from build123d import *

# Parameters (mm, degrees)
TALADRO_DE_MARGEN_PARA_1_41_D = 6.7564


with BuildPart() as part:
    # Croquis2 → Revolución1 (revolve)
    with BuildSketch(Plane.XY, mode=Mode.PRIVATE) as revoluci_n1_sk:
        Polygon((9.5, 37.5), (9.5, -37.5), (13.5, -37.5), (13.5, -7.5), (25.4, -7.5), (25.4, 7.5), (13.5, 7.5), (13.5, 37.5), align=None)
    revolve(revoluci_n1_sk.sketch.rotate(Axis((0, 0, 0), (0, -1, 0)), 90), axis=Axis((0, 0, 0), (0, -1, 0)))

    # Taladro de margen para 1/41 (through all)
    with Locations(Plane(origin=(0, 7.5, 0), x_dir=(1, 0, 0), z_dir=(0, 1, 0))):
        with Locations((19.45, 0), (-19.45, 0)):
            Hole(TALADRO_DE_MARGEN_PARA_1_41_D / 2)


solid = part.part
Source: CAD feature listing. Evaluate the final solid. Frame: model axes, mm. A direction names the side the tool comes from. Round coordinates to 2 decimals unless told otherwise and drop trailing zeros. Loops run counter-clockwise (first coordinate to the right, second up) from the corner with the lowest first, then second, coordinate; pieces in that order, holes last. Notation, with made-up numbers: (84.25, 39) - (95.25, 39) arc R9 cw to (95.25, 55) - close; hole circle Ø6 at (47, -17). An arc over 180 degrees is marked (long way). Write item = value, one per line. Start each with the question number.
(1) Pin query (flat end, axial travel): pin 1 (3 mm diameter, centred on y = 0.5, z = 20, fed in from +X); pin 2 (10 mm diameter, centred on x = -1.5, y = 17.5, fed in from -Z); pin 3 (8 mm diameter, centred on x = 19.45, z = 0, fed in from -Y); pin 4 (8 mm diameter, centred on x = 2.5, z = 7.5, fed in from -Y). Return the tip coordinate at first contact, or that it passes through.
(2) Pull-direction query (Z, two-part tool) for faces 4 (the face through (13.18, -22.29, -2.93)), 5 (the face through (-9.2, 37.5, -3.2)), 6 (the face through (-22.571, -0.105, 1.294)); classes: +Z half, -Z half, draft (parallel to the pull), parting line (faces both ways), or undercut.
(3) Section query B-B, the plane z = 0. Output: boundary loops of the cut face in (x, y).
(4) Section query A-A, the plane x = 0. Output: boundary loops of the cut face in (y, z), plus the area to 3 significant figures.
(5) Section query D-D, the plane y = -2.5. Output: boundary loops of the cut face in (x, z), plus the area to 3 significant figures.
(6) Ray query, line 1 along X through (y, z) = (-11, 0); line 2 along Z through (x, y) = (-5.5, 4.5); line 3 along Y through (x, z) = (-20.5, 8). Return the intervals inside material, ascending. Write a range as from..to.
(7) Set-up query: faces 1 (the face through (16.329, -0.105, 1.294)), 2 (the face through (11, -7.5, -11)), 3 (the face through (13.18, 22.71, -2.93)). Return all of +Z, -Z, +X, -X, +Y, -Y with unobstructed straight access to the full face (end or side cutting, diameter ignored); none if empty.
(8) Section query C-C, the plane y = 11. Output: boundary loops of the cut face in (x, z), plus the area to 3 significant figures.
Conclusion:
q1.pin_1 = 17.4
q1.pin_2 = -13.5
q1.pin_3 = -7.5
q1.pin_4 = -37.5
q2.face_4 = parting line
q2.face_5 = draft
q2.face_6 = undercut
q3.outline = (-25.4, -7.5) - (-22.83, -7.5) - (-22.83, 7.5) - (-25.4, 7.5) - close; (-16.07, -7.5) - (-13.5, -7.5) - (-13.5, -37.5) - (-9.5, -37.5) - (-9.5, 37.5) - (-13.5, 37.5) - (-13.5, 7.5) - (-16.07, 7.5) - close; (9.5, -37.5) - (13.5, -37.5) - (13.5, -7.5) - (16.07, -7.5) - (16.07, 7.5) - (13.5, 7.5) - (13.5, 37.5) - (9.5, 37.5) - close; (22.83, -7.5) - (25.4, -7.5) - (25.4, 7.5) - (22.83, 7.5) - close
q4.outline = (-37.5, -13.5) - (-7.5, -13.5) - (-7.5, -25.4) - (7.5, -25.4) - (7.5, -13.5) - (37.5, -13.5) - (37.5, -9.5) - (-37.5, -9.5) - close; (-37.5, 9.5) - (37.5, 9.5) - (37.5, 13.5) - (7.5, 13.5) - (7.5, 25.4) - (-7.5, 25.4) - (-7.5, 13.5) - (-37.5, 13.5) - close
q4.area = 957 mm2
q5.outline = circle Ø50.8 at (0, 0); hole circle Ø6.76 at (-19.45, 0); hole circle Ø19 at (0, 0); hole circle Ø6.76 at (19.45, 0)
q5.area = 1,670 mm2
q6.line_1 = -13.5..-9.5, 9.5..13.5
q6.line_2 = -24.8..-7.75, 7.75..24.8
q6.line_3 = -7.5..7.5
q7.face_1 = +Y, -Y
q7.face_2 = -Y
q7.face_3 = +Y
q8.outline = circle Ø27 at (0, 0); hole circle Ø19 at (0, 0)
q8.area = 289 mm2
